Verification items for the finished model (mm, model axes). Give positions to 0.01 mm unless a question says otherwise; leave off trailing zeros. Loops run counter-clockwise (first coordinate to the right, second up) from the corner with the lowest first, then second, coordinate; pieces in that order, holes last. Notation, with made-up numbers: M 53.5,34 L 58.5,34 A25 ccw 58.5,65 Z; hole C -4,60.25 d10. An arc over 180 degrees is marked long. Put each result on its own line as item: value. Start each with the question number.
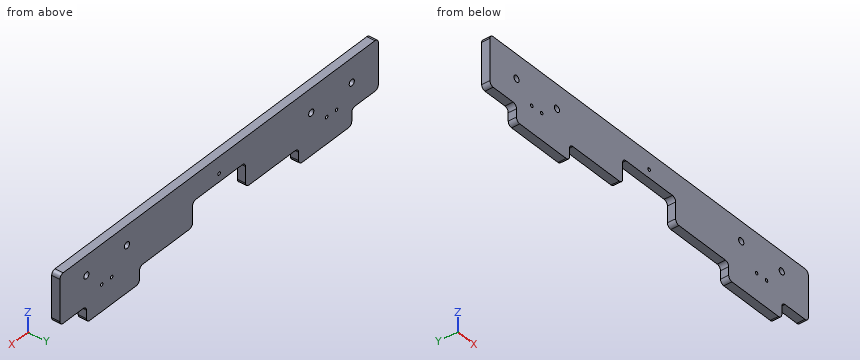
from build123d import *

# Parameters (mm, degrees)
SKETCH1_W           = 304.8
SKETCH1_H           = 38.1
BOSS_EXTRUDE1_DEPTH = 6.35
SKETCH5_W           = 50.8
SKETCH5_H           = 12.7
BOSS_EXTRUDE2_DEPTH = 6.35
FILLET1_R           = 3.175
FILLET2_R           = 3.175
SKETCH2_R           = 1.4732
CUT_EXTRUDE1_DEPTH  = 6.35
SKETCH3_R           = 1.2
CUT_EXTRUDE2_DEPTH  = 6.35
SKETCH4_R           = 2.4765
CUT_EXTRUDE3_DEPTH  = 6.35
SKETCH6_W           = 50.8
SKETCH6_H           = 19.05
CUT_EXTRUDE4_DEPTH  = 6.35
FILLET3_R           = 3.175
SKETCH7_R           = 1.2192
CUT_EXTRUDE5_DEPTH  = 6.35


with BuildPart() as part:
    # Sketch1 → Boss-Extrude1 (new body)
    with BuildSketch(Plane(origin=(0, 0, 0), x_dir=(1, 0, 0), z_dir=(0, 1, 0))):
        Rectangle(SKETCH1_W, SKETCH1_H)
    extrude(amount=BOSS_EXTRUDE1_DEPTH)

    # Sketch5 → Boss-Extrude2 (add)
    with BuildSketch(Plane(origin=(0, 6.35, 0), x_dir=(1, 0, 0), z_dir=(0, 1, 0))):
        with Locations((-101.6, 25.4)):
            Rectangle(SKETCH5_W, SKETCH5_H)
        with Locations((101.6, 25.4)):
            Rectangle(SKETCH5_W, SKETCH5_H)
    extrude(amount=-BOSS_EXTRUDE2_DEPTH)

    # Fillet1
    fillet1_edges = [part.edges().sort_by_distance(p)[0] for p in [
        (127, 3.175, -19.05),
        (127, 3.175, -31.75),
        (76.2, 3.175, -31.75),
        (76.2, 3.175, -19.05),
        (-76.2, 3.175, -19.05),
        (-76.2, 3.175, -31.75),
        (-127, 3.175, -31.75),
        (-127, 3.175, -19.05),
    ]]
    fillet(fillet1_edges, radius=FILLET1_R)

    # Fillet2
    fillet2_edges = [part.edges().sort_by_distance(p)[0] for p in [
        (152.4, 3.175, -19.05),
        (152.4, 3.175, 19.05),
        (-152.4, 3.175, 19.05),
        (-152.4, 3.175, -19.05),
    ]]
    fillet(fillet2_edges, radius=FILLET2_R)

    # Sketch2 → Cut-Extrude1 (cut)
    with BuildSketch(Plane(origin=(0, 6.35, 0), x_dir=(1, 0, 0), z_dir=(0, 1, 0))):
        with Locations((0, 12.7)):
            Circle(SKETCH2_R)
    extrude(amount=-CUT_EXTRUDE1_DEPTH, mode=Mode.SUBTRACT)

    # Sketch3 → Cut-Extrude2 (cut)
    with BuildSketch(Plane(origin=(0, 6.35, 0), x_dir=(1, 0, 0), z_dir=(0, 1, 0))):
        with Locations((-112.4, 11.35)):
            Circle(SKETCH3_R)
        with Locations((-102.9, 11.35)):
            Circle(SKETCH3_R)
    cut_extrude2 = extrude(amount=-CUT_EXTRUDE2_DEPTH, mode=Mode.SUBTRACT)

    # Mirror1: Cut-Extrude2 across plane
    add(cut_extrude2.mirror(Plane(origin=(0, 0, 0), x_dir=(0, 0, 1), z_dir=(1, 0, 0))), mode=Mode.SUBTRACT)

    # Sketch4 → Cut-Extrude3 (cut)
    with BuildSketch(Plane(origin=(0, 6.35, 0), x_dir=(1, 0, 0), z_dir=(0, 1, 0))):
        with Locations((-127, -0.457547173)):
            Circle(SKETCH4_R)
        with Locations((-88.2, -0.457547173)):
            Circle(SKETCH4_R)
        with Locations((88.2, -4.001229652)):
            Circle(SKETCH4_R)
        with Locations((127, -4.001229652)):
            Circle(SKETCH4_R)
    extrude(amount=-CUT_EXTRUDE3_DEPTH, mode=Mode.SUBTRACT)

    # Sketch6 → Cut-Extrude4 (cut)
    with BuildSketch(Plane(origin=(0, 6.35, 0), x_dir=(1, 0, 0), z_dir=(0, 1, 0))):
        with Locations((0, 9.525)):
            Rectangle(SKETCH6_W, SKETCH6_H)
    extrude(amount=-CUT_EXTRUDE4_DEPTH, mode=Mode.SUBTRACT)

    # Fillet3
    fillet3_edges = [part.edges().sort_by_distance(p)[0] for p in [
        (25.4, 3.175, -19.05),
        (25.4, 3.175, 0),
        (-25.4, 3.175, 0),
        (-25.4, 3.175, -19.05),
    ]]
    fillet(fillet3_edges, radius=FILLET3_R)

    # Sketch7 → Cut-Extrude5 (cut)
    with BuildSketch(Plane(origin=(0, 6.35, 0), x_dir=(1, 0, 0), z_dir=(0, 1, 0))):
        with Locations((0, -6.35)):
            Circle(SKETCH7_R)
    extrude(amount=-CUT_EXTRUDE5_DEPTH, mode=Mode.SUBTRACT)


solid = part.part
Q1. Cross-section at C-C, the plane y = 1.75. State how many separate pieces and enclosed holes the cut face has, then the cut area to 3 significant figures.
Q2. Go/stop test with flat-tipped pins: pin 1 (3 mm diameter, centred on x = -137, y = 4.5, fed in from -Z); pin 2 (3 mm diameter, centred on y = 4, z = -24, fed in from +X); pin 3 (4 mm diameter, centred on x = -88.2, z = 0.46, fed in from -Y) (1 decimal); pin 4 (1.9 mm diameter, centred on y = 3.5, z = -24.5, fed in from -X). Record where each tip stops, or that it passes through.
Q3. Cross-section at A-A, the plane x = -88.2. Record the boundary of the cut face in (y, z).
Q4. Scan lines: L1, parallel to X at y = 1.5, z = -11.35; L2, parallel to X at y = 3, z = -24; L3, parallel to X at y = 2.75, z = -15. Record each from-to range of solid material in increasing order.
Q5. Cross-section at B-B, the plane x = -53. Record the boundary of the cut face in (y, z), then the cut area to 3 significant figures.
Ans:
1. separate pieces: 1
1. enclosed holes: 9
1. area: 11,800 mm^2
2. pin 1: stops at z = -19.05
2. pin 2: stops at x = 127
2. pin 3: passes through
2. pin 4: stops at x = -127
3. outline: M 0,-31.75 L 6.35,-31.75 L 6.35,-2.02 L 0,-2.02 Z; M 0,2.93 L 6.35,2.93 L 6.35,19.05 L 0,19.05 Z
4. L1: x = -152.4 to -113.6, -111.2 to -104.1, -101.7 to -25.4, 25.4 to 101.7, 104.1 to 111.2, 113.6 to 152.4
4. L2: x = -127 to -76.2, 76.2 to 127
4. L3: x = -152.4 to -25.4, 25.4 to 152.4
5. outline: M 0,-19.05 L 6.35,-19.05 L 6.35,19.05 L 0,19.05 Z
5. area: 242 mm^2
